Geometry check sheet. Reference: drawing and pictorial views, mm from the part's lowest x, y, z. Give positions to 0.01 mm unless a question says otherwise; leave off trailing zeros. Order: outer loops, then holes, each group sorted by start corner. A loop starts at its lowest first (then second) coordinate and runs counter-clockwise, first axis right, second up. Notation, with made-up numbers: (21, 66.25) - (59, 66.25) arc R7 ccw to (59, 75.25) - close; hole circle Ø4 at (87, 78.25). An arc over 180 degrees is marked (long way). Answer as a JSON object with one key per item and string values.
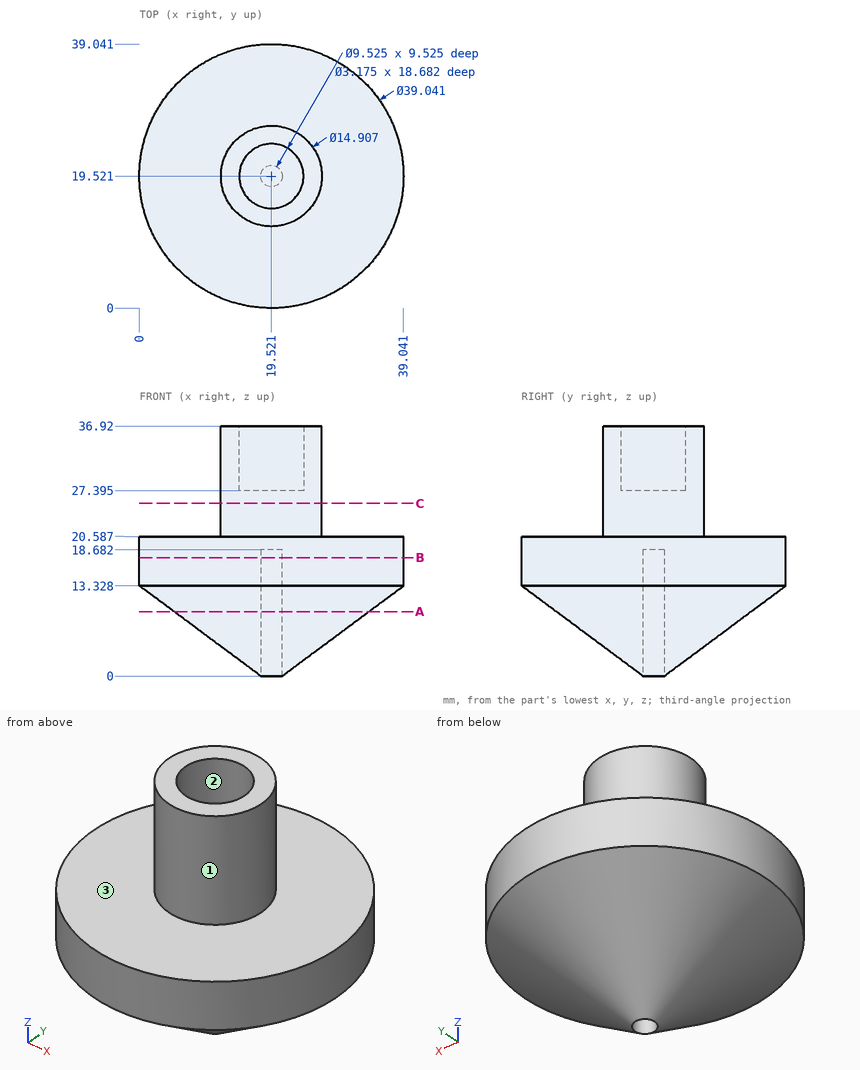
(1) Release check for a two-part mould opening along X. For the marked faces 1, 2 and 3 record: pulls with the +X half, pulls with the -X half, needs draft (parallel to the pull), parting line crosses it, or undercut.
Computed values:
{"face 1": "parting line crosses it", "face 2": "undercut", "face 3": "needs draft"}
(2) Section check A-A (z = 9.5). Record the cut outline in (x, y) (1 decimal).
Computed values:
{"outline": "circle Ø28.7 at (19.5, 19.5); hole circle Ø3.2 at (19.5, 19.5)"}
(3) Gauge pin test, flat ends, axial feed: pin 1 Ø3 at (x, y) = (17.5, 19.5) entering from +Z (1 decimal); pin 2 Ø4 at (x, z) = (17.5, 26.5) entering from -Y; pin 3 Ø12 at (x, y) = (31.5, 11.5) entering from -Z (1 decimal). Record the tip position at first contact, or that the pin passes through.
Computed values:
{"pin 1": "stops at z = 27.4", "pin 2": "stops at y = 12.07", "pin 3": "stops at z = 5.1"}
(4) Section check C-C (z = 25.5). Record the cut outline in (x, y).
Computed values:
{"outline": "circle Ø14.91 at (19.52, 19.52)"}
(5) Section check B-B (z = 17.5). Record the cut outline in (x, y) (1 decimal).
Computed values:
{"outline": "circle Ø39 at (19.5, 19.5); hole circle Ø3.2 at (19.5, 19.5)"}
(6) Material ranges on line 1 along X through (y, z) = (23, 30) (1 decimal); line 2 along X through (y, z) = (22.5, 33.5) (1 decimal); line 3 along Y through (x, z) = (13, 23), recorded low to high. Write a range as [from, to].
Computed values:
{"line 1": "x = [12.9, 16.3], [22.8, 26.1]", "line 2": "x = [12.7, 15.8], [23.2, 26.4]", "line 3": "y = [15.91, 23.13]"}
